from build123d import *

# Parameters (mm, degrees)
ESQUISSE2_W             = 12.1
ESQUISSE2_H             = 10.1
ENL_V_MAT_EXTRU_1_DEPTH = 21.3
ESQUISSE3_R             = 1.55
ENL_V_MAT_EXTRU_2_DEPTH = 21.3
ESQUISSE5_R             = 4.25
ENL_V_MAT_EXTRU_3_DEPTH = 21.3


with BuildPart() as part:
    # Esquisse1 → Révolution1 (revolve)
    with BuildSketch(Plane.XY):
        Polygon((0, 0), (40, 0), (40, 19), (50, 19), (50, 22), (40, 22), (0, 22), align=None)
    revolve(axis=Axis((0, 0, 0), (0, 1, 0)))

    # Esquisse2 → Enlèv. mat.-Extru.1 (cut)
    with BuildSketch(Plane(origin=(0, 22, 0), x_dir=(1, 0, 0), z_dir=(0, 1, 0))):
        Rectangle(ESQUISSE2_W, ESQUISSE2_H)
    extrude(amount=-ENL_V_MAT_EXTRU_1_DEPTH, mode=Mode.SUBTRACT)

    # Esquisse3 → Enlèv. mat.-Extru.2 (cut)
    with BuildSketch(Plane(origin=(0, 22, 0), x_dir=(1, 0, 0), z_dir=(0, 1, 0))):
        with Locations(Location((45, 0, 0), (0, 0, 180))):
            Circle(ESQUISSE3_R)
        with Locations((-45, 0)):
            Circle(ESQUISSE3_R)
        with Locations(Location((0, 45, 0), (0, 0, 180))):
            Circle(ESQUISSE3_R)
        with Locations((0, -45)):
            Circle(ESQUISSE3_R)
    extrude(amount=-ENL_V_MAT_EXTRU_2_DEPTH, mode=Mode.SUBTRACT)

    # Esquisse5 → Enlèv. mat.-Extru.3 (cut)
    with BuildSketch(Plane(origin=(0, 0.7, 0), x_dir=(1, 0, 0), z_dir=(0, 1, 0))):
        with Locations(Location((0, 0, 0), (0, 0, 180))):
            Circle(ESQUISSE5_R)
    extrude(amount=-ENL_V_MAT_EXTRU_3_DEPTH, mode=Mode.SUBTRACT)


solid = part.part
Can you work these out from the model? Positions are in its coordinate system, mm. A direction names the side the tool comes from. Round coordinates to 2 decimals unless told otherwise and drop trailing zeros. Order: outer loops, then holes, each group sorted by start corner. A loop starts at its lowest first (then second) coordinate and runs counter-clockwise, first axis right, second up. Notation, with made-up numbers: (39.25, -31) -> (70.25, -31) arc R11 ccw to (70.25, -17) -> close; hole circle Ø11 at (76.25, 39.25). An arc over 180 degrees is marked (long way). Write each question's results on one line, items separated by ' | '. Start each with the question number.
Item 1: Please list where these lines run through material, in increasing order: L1, parallel to Z at x = 0, y = 20.5; L2, parallel to Z at x = 0, y = 0.25; L3, parallel to Z at x = -3, y = 2.5.
Item 2: Will these pins go through, and if not, where does the flat tip stop? pin 1 (10 mm diameter, centred on x = 0, z = 0, fed in from +Y); pin 2 (4 mm diameter, centred on y = 10, z = 22, fed in from +X); pin 3 (5 mm diameter, centred on x = 0, z = 45, fed in from -Y); pin 4 (5 mm diameter, centred on x = -20, z = 36, fed in from -Y).
Item 3: Thinking about a two-plate mould opening in Z: for faces 4 (the flat face through (6.05, 11, 0)), 5 (the flat face through (0, 11, 5.05)), 6 (the flat face through (-1, 22, 10)), 7 (the cylindrical face through (-8.67, 9.63, 39.05)), which applies, +Z half, -Z half, draft (parallel to the pull), parting line (faces both ways), or undercut?
Item 4: If we section it at C-C, the plane y = 7: Write out the boundary of the cut face in (x, z).
Item 5: If we section it at A-A, the plane x = 0: Write out the boundary of the cut face in (y, z).
Item 6: If we section it at B-B, the plane z = 45: Write out the boundary of the cut face in (x, y).
Item 7: If we section it at D-D, the plane x = -45: Write out the boundary of the cut face in (y, z), then the cut area to 3 significant figures.
Item 8: Which directions (+Z, -Z, +X, -X, +Y, -Y) give clear straight access to the entire face, cutting with the end or side of a thin tool? Please do faces 1 (the flat face through (15, 19, -37.3)), 2 (the flat face through (-8, 0, -1)), 3 (the flat face through (0, 11, -5.05)).
Results:
1) L1: z = -50 to -46.55, -43.45 to -5.05, 5.05 to 43.45, 46.55 to 50 | L2: z = -40 to -4.25, 4.25 to 40 | L3: z = -39.89 to -5.05, 5.05 to 39.89
2) pin 1: stops at y = 0.7 | pin 2: stops at x = 34.64 | pin 3: stops at y = 19 | pin 4: stops at y = 0
3) face 4: undercut | face 5: undercut | face 6: draft | face 7: parting line
4) outline: circle Ø80 at (0, 0); hole (-6.05, -5.05) -> (6.05, -5.05) -> (6.05, 5.05) -> (-6.05, 5.05) -> close
5) outline: (0, -40) -> (19, -40) -> (19, -43.45) -> (22, -43.45) -> (22, -5.05) -> (0.7, -5.05) -> (0.7, -4.25) -> (0, -4.25) -> close; (0, 4.25) -> (0.7, 4.25) -> (0.7, 5.05) -> (22, 5.05) -> (22, 43.45) -> (19, 43.45) -> (19, 40) -> (0, 40) -> close; (19, -50) -> (22, -50) -> (22, -46.55) -> (19, -46.55) -> close; (19, 46.55) -> (22, 46.55) -> (22, 50) -> (19, 50) -> close
6) outline: (-21.79, 19) -> (-1.55, 19) -> (-1.55, 22) -> (-21.79, 22) -> close; (1.55, 19) -> (21.79, 19) -> (21.79, 22) -> (1.55, 22) -> close
7) outline: (19, -21.79) -> (22, -21.79) -> (22, -1.55) -> (19, -1.55) -> close; (19, 1.55) -> (22, 1.55) -> (22, 21.79) -> (19, 21.79) -> close | area: 121 mm2
8) face 1: -Y | face 2: +Z, -Z, +X, -X, -Y | face 3: +Y
